Source: CAD feature listing. Evaluate the final solid. Frame: model axes, mm. Face numbers are marked on the shaded views. A direction names the side the tool comes from. Coordinates: 2 decimals unless noted, no trailing zeros. Loops run counter-clockwise (first coordinate to the right, second up) from the corner with the lowest first, then second, coordinate; pieces in that order, holes last.
Item 1: Section query B-B, the plane x = 29. Return the cut outline in (y, z), then the cut area to 3 significant figures.
Item 2: Section query D-D, the plane y = 20.5. Return the cut outline in (x, z), then the cut area to 3 significant figures.
Item 3: Section query C-C, the plane z = 0.75. Return the cut outline in (x, y), then the cut area to 3 significant figures.
Item 4: Reachability of the marked faces 1, 2, 3 and 4 from +Z, -Z, +X, -X, +Y, -Y: full face, straight path, thin tool, end or side. Return the list, or none.
Item 5: Line query: probe 1 along Y at (x, z) = (11, 0.2); probe 2 along X at (y, z) = (11.5, 1.5); probe 3 along Y at (x, z) = (18, 1.05). Output: solid intervals per line, ascending.
Item 6: Pull-direction query (X, two-part tool) for the marked faces 5, 6 and 7; classes: +X half, -X half, draft (parallel to the pull), parting line (faces both ways), or undercut.
Item 7: Pin query (flat end, axial travel): pin 1 Ø1 at (x, z) = (8, 1) entering from -Y; pin 2 Ø2 at (x, y) = (34, 26) entering from +Z (3 decimals); pin 3 Ø1 at (x, z) = (27, 2) entering from +Y. Return the tip coordinate at first contact, or that it passes through.
Item 8: Section query A-A, the plane y = 40. Return the cut outline in (x, z).
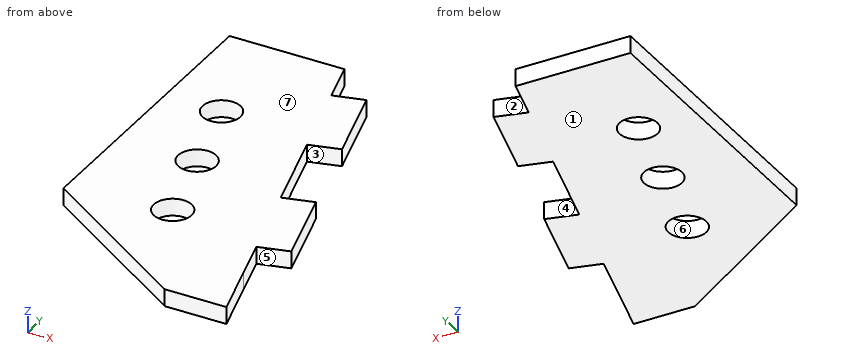
```python
from build123d import *

# Parameters (mm, degrees)
RESSALTO_EXTRUS_O1_DEPTH = 3
FURO_COM_FOLGA_DE_M61_D  = 6.6
RESSALTO_EXTRUS_O2_DEPTH = 3
RESSALTO_EXTRUS_O3_DEPTH = 3
CORTE_EXTRUS_O1_DEPTH    = 72.798210781


with BuildPart() as part:
    # Esboço1 → Ressalto-extrusão1 (new body)
    with BuildSketch(Plane.XY):
        Polygon((0, 0), (0, 60), (20, 60), (36.076951546, 0), align=None)
    extrude(amount=RESSALTO_EXTRUS_O1_DEPTH)

    # Furo com folga de M61 (through all)
    with Locations(Plane.XY.offset(3)):
        with Locations((9.829841142, 40), (13.712126819, 25.511112606), (17.594412496, 11.022225211)):
            Hole(FURO_COM_FOLGA_DE_M61_D / 2)

    # Esboço4 → Ressalto-extrusão2 (add)
    with BuildSketch(Plane.XY.offset(3)):
        Polygon((22.070552361, 52.27259339), (27.383144405, 53.696098138), (31.265430082, 39.207210743), (25.952838037, 37.783705995), align=None)
        Polygon((30.124113509, 22.216294005), (35.436705553, 23.639798753), (39.31899123, 9.150911358), (34.006399185, 7.72740661), align=None)
    extrude(amount=-RESSALTO_EXTRUS_O2_DEPTH)

    # Esboço5 → Ressalto-extrusão3 (add)
    with BuildSketch(Plane.XY.offset(3)):
        Polygon((0, 0), (0, -10), (38.75644347, -10), (36.076951546, 0), align=None)
    extrude(amount=-RESSALTO_EXTRUS_O3_DEPTH)

    # Esboço6 → Corte-extrusão1 (cut, through all)
    with BuildSketch(Plane.XY.offset(3)):
        Polygon((0, 8.5), (0, -10), (28, -10), align=None)
    extrude(amount=-CORTE_EXTRUS_O1_DEPTH, mode=Mode.SUBTRACT)


solid = part.part
```
Verdict:
1. outline: (-10, 0) - (26.41, 0) - (26.41, 3) - (-10, 3) - close; (38.6, 0) - (47.66, 0) - (47.66, 3) - (38.6, 3) - close
1. area: 136 mm2
2. outline: (0, 0) - (36.28, 0) - (36.28, 3) - (0, 3) - close
2. area: 109 mm2
3. outline: (0, 8.5) - (28, -10) - (38.76, -10) - (34.01, 7.73) - (39.32, 9.15) - (35.44, 23.64) - (30.12, 22.22) - (25.95, 37.78) - (31.27, 39.21) - (27.38, 53.7) - (22.07, 52.27) - (20, 60) - (0, 60) - close; hole circle Ø6.6 at (9.83, 40); hole circle Ø6.6 at (13.71, 25.51); hole circle Ø6.6 at (17.59, 11.02)
3. area: 1,860 mm2
4. face 1: -Z, +X, -X, +Y, -Y
4. face 2: +Z, -Z, +Y
4. face 3: +Z, -Z, +X
4. face 4: +Z, -Z
5. probe 1: y = 1.23 to 23.63, 27.39 to 36.91, 43.09 to 60
5. probe 2: x = 0 to 14.33, 20.86 to 38.69
5. probe 3: y = -3.39 to 7.75, 14.3 to 60
6. face 5: +X half
6. face 6: undercut
6. face 7: draft
7. pin 1: stops at y = 2.88
7. pin 2: passes through
7. pin 3: stops at y = 53.7
8. outline: (0, 0) - (6.53, 0) - (6.53, 3) - (0, 3) - close; (13.13, 0) - (31.05, 0) - (31.05, 3) - (13.13, 3) - close
